from build123d import *

# Parameters (mm, degrees)
SKETCH1_R      = 110
EXTRUDE1_DEPTH = 70
FILLET1_R      = 35
EXTRUDE2_DEPTH = 171.587221092
SKETCH3_R      = 5
EXTRUDE3_DEPTH = 171.587221262
EXTRUDE7_DEPTH = 2.5


# Read off the part's stored shape, not the designer's step: Shell1
with BuildPart() as part:
    # Sketch1 → Extrude1 (new body)
    with BuildSketch(Plane.XY):
        Circle(SKETCH1_R)
    extrude(amount=EXTRUDE1_DEPTH)

    # Fillet1
    fillet1_edges = [part.edges().sort_by_distance(p)[0] for p in [
        (-110, 0, 0),
        (-110, 0, 70),
    ]]
    fillet(fillet1_edges, radius=FILLET1_R - 0.0001)  # a hair under: the kernel refuses the full size

    # Sketch2 → Extrude2 (cut, through all)
    with BuildSketch(Plane.XY):
        with BuildLine():
            Line((43.301270189, 0), (110, 0))
            Line((110, 0), (110, -110))
            Line((110, -110), (-110, -110))
            Line((-110, -110), (-110, 0))
            Line((-110, 0), (-43.301270189, 0))
            ThreePointArc((-43.301270189, 0), (-30.801270189, -3.349364905), (-21.650635095, -12.5))
            ThreePointArc((-21.650635095, -12.5), (0, -25), (21.650635095, -12.5))
            ThreePointArc((21.650635095, -12.5), (30.801270189, -3.349364905), (43.301270189, 0))
        make_face()
    extrude(amount=EXTRUDE2_DEPTH, mode=Mode.SUBTRACT)

    # Shell1 outline → Shell1 (revolve, cut)
    with BuildSketch(Plane.XZ):
        with BuildLine():
            Line((0, 65), (0, 5))
            Line((0, 5), (75, 5))
            ThreePointArc((75, 5), (96.213203436, 13.786796564), (105, 35))
            ThreePointArc((105, 35), (96.213203436, 56.213203436), (75, 65))
            Line((75, 65), (0, 65))
        make_face()
    revolve(axis=Axis((0, 0, 0), (0, 0, 1)), mode=Mode.SUBTRACT)

    # Sketch3 → Extrude3 (cut, through all)
    with BuildSketch(Plane.XY.offset(70)):
        Circle(SKETCH3_R)
    extrude(amount=-EXTRUDE3_DEPTH, mode=Mode.SUBTRACT)

    # Sketch5 → Extrude7 (cut)
    with BuildSketch(Plane.XY.offset(70)):
        with BuildLine():
            Line((-27.271780287, 2.5), (-48.412291828, 2.5))
            ThreePointArc((-48.412291828, 2.5), (-56.317985978, 6.376275643), (-58.094750193, 15))
            ThreePointArc((-58.094750193, 15), (-51.961524227, 30), (-42.037756153, 42.811529494))
            ThreePointArc((-42.037756153, 42.811529494), (-33.681009677, 45.584668725), (-26.371209423, 40.676274578))
            Line((-26.371209423, 40.676274578), (-15.800953653, 22.368054535))
            ThreePointArc((-15.800953653, 22.368054535), (-14.472209198, 16.899109859), (-16.307471794, 11.578703023))
            ThreePointArc((-16.307471794, 11.578703023), (-17.320508076, 10), (-18.181186858, 8.333333333))
            ThreePointArc((-18.181186858, 8.333333333), (-21.871163038, 4.083745885), (-27.271780287, 2.5))
        make_face()
        with BuildLine():
            Line((-11.470826634, 24.868054535), (-22.041082404, 43.176274578))
            ThreePointArc((-22.041082404, 43.176274578), (-22.636976301, 51.960944368), (-16.05699404, 57.811529494))
            ThreePointArc((-16.05699404, 57.811529494), (0, 60), (16.05699404, 57.811529494))
            ThreePointArc((16.05699404, 57.811529494), (22.636976301, 51.960944368), (22.041082404, 43.176274578))
            Line((22.041082404, 43.176274578), (11.470826634, 24.868054535))
            ThreePointArc((11.470826634, 24.868054535), (7.39895384, 20.982855743), (1.873715064, 19.912036356))
            ThreePointArc((1.873715064, 19.912036356), (0, 20), (-1.873715064, 19.912036356))
            ThreePointArc((-1.873715064, 19.912036356), (-7.39895384, 20.982855743), (-11.470826634, 24.868054535))
        make_face()
        with BuildLine():
            Line((27.271780287, 2.5), (48.412291828, 2.5))
            ThreePointArc((48.412291828, 2.5), (56.317985978, 6.376275643), (58.094750193, 15))
            ThreePointArc((58.094750193, 15), (51.961524227, 30), (42.037756153, 42.811529494))
            ThreePointArc((42.037756153, 42.811529494), (33.681009677, 45.584668725), (26.371209423, 40.676274578))
            Line((26.371209423, 40.676274578), (15.800953653, 22.368054535))
            ThreePointArc((15.800953653, 22.368054535), (14.472209198, 16.899109859), (16.307471794, 11.578703023))
            ThreePointArc((16.307471794, 11.578703023), (17.320508076, 10), (18.181186858, 8.333333333))
            ThreePointArc((18.181186858, 8.333333333), (21.871163038, 4.083745885), (27.271780287, 2.5))
        make_face()
    extrude(amount=-EXTRUDE7_DEPTH, mode=Mode.SUBTRACT)


solid = part.part
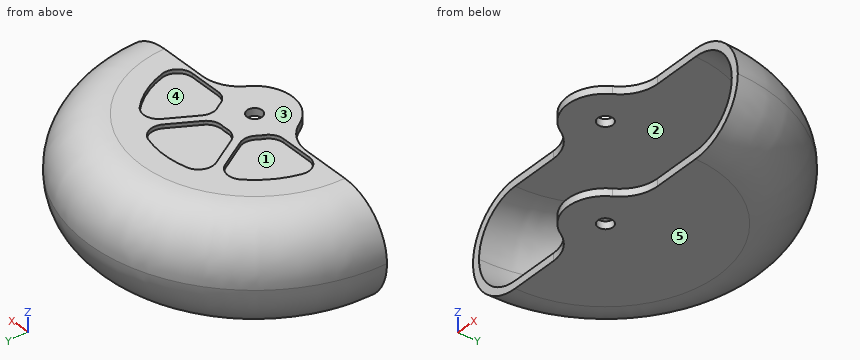
Geometry: final body of the model. Coordinates: model frame, mm. Face numbers are marked on the shaded views. A direction names the side the tool comes from. Give positions to 0.01 mm unless a question says otherwise; leave off trailing zeros. Loops run counter-clockwise (first coordinate to the right, second up) from the corner with the lowest first, then second, coordinate; pieces in that order, holes last. Notation, with made-up numbers: M -17.75,44.25 L -11.75,44.25 A38 ccw -11.75,83.25 Z; hole C 34.5,-27 d3. An arc over 180 degrees is marked long. Put each result on its own line as item: value.
1) Mould query, pull axis X, two halves, no side actions, for the marked faces 4 and 5. Classes: released by +X, released by -X, zero draft, split by the parting line, or undercut.
Computed values:
face 4: undercut
face 5: zero draft
2) Cut plane A-A, the plane z = 40. Return the cut outline in (x, y).
Computed values:
outline: M -109.64,0 L -104.58,0 A104.58 cw 104.58,0 L 109.64,0 A109.64 ccw Z
3) Material intervals for L1, parallel to Z at x = 29.5, y = 41.5; L2, parallel to Z at x = 87, y = 11.5; L3, parallel to X at y = 66, z = 29.5, sorted ascending. Write a range as from..to.
Computed values:
L1: z = 0..5, 65..67.5
L2: z = 2.41..7.85, 62.15..67.59
L3: x = -87.46..-81.01, 81.01..87.46
4) First-contact query: P1, Ø2, axis at x = 44, z = 23.5, coming from the +Y side; P2, Ø5, axis at x = 21.5, z = 36.5, coming from the -Y side; P3, Ø1.5, axis at x = 16, y = 76, coming from the -Z side. Flat tips, straight axial feed; report the tip coordinate or a pass-through.
Computed values:
P1: stops at y = 99.27
P2: stops at y = 102.16
P3: stops at z = 0.05
5) Reachability of the marked faces 1, 2 and 3 from +Z, -Z, +X, -X, +Y, -Y: full face, straight path, thin tool, end or side. Return the list, or none.
Computed values:
face 1: +Z
face 2: -Y
face 3: +Z, +X, -X, +Y, -Y
6) Cut plane B-B, the plane z = 18. Return the cut outline in (x, y), plus the area to 3 significant figures.
Computed values:
outline: M -105.59,0 L -99.72,0 A99.72 cw 99.72,0 L 105.59,0 A105.59 ccw Z
area: 1,890 mm^2
